from build123d import *

# Parameters (mm, degrees)
SKETCH_1_W          = 40
SKETCH_1_H          = 20
EXTRUDE_1_DEPTH     = 149.5
SKETCH_2_W          = 38
SKETCH_2_H          = 18
CUT_EXTRUDE_1_DEPTH = 2999
SKETCH_4_R          = 2.05
CUT_EXTRUDE_2_DEPTH = 2999
SKETCH_5_R          = 2.025
CUT_EXTRUDE_3_DEPTH = 2999
CUT_EXTRUDE_START   = -21
SKETCH_6_R          = 1.525
CUT_EXTRUDE_4_DEPTH = 22
CUT_EXTRUDE_START_2 = -41
SKETCH_8_R          = 1.525
CUT_EXTRUDE_5_DEPTH = 42


with BuildPart() as part:
    # 草图1 → 凸台-拉伸1 (new body, symmetric)
    with BuildSketch(Plane(origin=(0, 0, 0), x_dir=(0, 0, -1), z_dir=(1, 0, 0))):
        Rectangle(SKETCH_1_W, SKETCH_1_H)
    extrude(amount=EXTRUDE_1_DEPTH, both=True)

    # 草图2 → 切除-拉伸1 (cut)
    with BuildSketch(Plane.ZY.offset(149.5)):
        Rectangle(SKETCH_2_W, SKETCH_2_H)
    extrude(amount=-CUT_EXTRUDE_1_DEPTH, mode=Mode.SUBTRACT)

    # 草图4 → 切除-拉伸2 (cut)
    with BuildSketch(Plane(origin=(0, 10, 0), x_dir=(1, 0, 0), z_dir=(0, 1, 0))):
        with Locations((-47.5, 12.5)):
            Circle(SKETCH_4_R)
        with Locations((-47.5, -12.5)):
            Circle(SKETCH_4_R)
        with Locations((47.5, 12.5)):
            Circle(SKETCH_4_R)
        with Locations((47.5, -12.5)):
            Circle(SKETCH_4_R)
    extrude(amount=-CUT_EXTRUDE_2_DEPTH, mode=Mode.SUBTRACT)

    # 草图5 → 切除-拉伸3 (cut)
    with BuildSketch(Plane.XZ.offset(10)):
        with Locations((-125.5, 14)):
            Circle(SKETCH_5_R)
        with Locations((-125.5, -14)):
            Circle(SKETCH_5_R)
        with Locations((-143.5, -14)):
            Circle(SKETCH_5_R)
        with Locations((-143.5, 14)):
            Circle(SKETCH_5_R)
    cut_extrude_3 = extrude(amount=-CUT_EXTRUDE_3_DEPTH, mode=Mode.SUBTRACT)

    # 镜向1: 切除-拉伸3 across plane
    add(cut_extrude_3.mirror(Plane(origin=(0, 0, 0), x_dir=(0, 0, 1), z_dir=(1, 0, 0))), mode=Mode.SUBTRACT)

    # 草图6 → 切除-拉伸4 (cut)
    with BuildSketch(Plane(origin=(0, 10, 0), x_dir=(1, 0, 0), z_dir=(0, 1, 0)).offset(CUT_EXTRUDE_START)):
        with Locations((-97.25, 16)):
            Circle(SKETCH_6_R)
        with Locations((-97.25, -16)):
            Circle(SKETCH_6_R)
        with Locations((-77.25, -16)):
            Circle(SKETCH_6_R)
        with Locations((-77.25, 16)):
            Circle(SKETCH_6_R)
    cut_extrude_4 = extrude(amount=CUT_EXTRUDE_4_DEPTH, mode=Mode.SUBTRACT)

    # 草图8 → 切除-拉伸5 (cut)
    with BuildSketch(Plane.XY.offset(20).offset(CUT_EXTRUDE_START_2)):
        with Locations((-107.25, 6)):
            Circle(SKETCH_8_R)
        with Locations((-87.25, 6)):
            Circle(SKETCH_8_R)
    cut_extrude_5 = extrude(amount=CUT_EXTRUDE_5_DEPTH, mode=Mode.SUBTRACT)

    # 镜向2: 切除-拉伸4, 切除-拉伸5 across plane
    add(cut_extrude_4.mirror(Plane(origin=(0, 0, 0), x_dir=(0, 0, 1), z_dir=(1, 0, 0))), mode=Mode.SUBTRACT)
    add(cut_extrude_5.mirror(Plane(origin=(0, 0, 0), x_dir=(0, 0, 1), z_dir=(1, 0, 0))), mode=Mode.SUBTRACT)


solid = part.part
Could you check a few things on this model? Use its own coordinates, in mm. A direction names the side the tool comes from. Give positions to 0.01 mm unless a question says otherwise; leave off trailing zeros. Loops run counter-clockwise (first coordinate to the right, second up) from the corner with the lowest first, then second, coordinate; pieces in that order, holes last. Notation, with made-up numbers: (9.5, 33) -> (53.5, 33) arc R17 ccw to (53.5, 48) -> close; hole circle Ø4 at (-33.5, 24.25). An arc over 180 degrees is marked (long way). Return JSON: item names as keys, results as strings.
Item 1: If we section it at C-C on x = 31: List the corners of the cut face in (y, z) for me.
Geometry results:
{"outline": "(-10, -20) -> (10, -20) -> (10, 20) -> (-10, 20) -> close; hole (-9, -19) -> (9, -19) -> (9, 19) -> (-9, 19) -> close"}
Item 2: If we section it at B-B on z = -7: List the corners of the cut face in (x, y) for me.
Geometry results:
{"outline": "(-149.5, -10) -> (149.5, -10) -> (149.5, -9) -> (-149.5, -9) -> close; (-149.5, 9) -> (149.5, 9) -> (149.5, 10) -> (-149.5, 10) -> close"}
Item 3: I need wall thicknesses on L1, parallel to Z at x = -47.5, y = -9.25; L2, parallel to Z at x = -125.5, y = -9.45 (3 decimals); L3, parallel to Y at x = -83.5, z = -10.5. Which ranges of each line are inside material? Lowest first, please. Write a range as from..to.
Geometry results:
{"L1": "z = -20..-14.55, -10.45..10.45, 14.55..20", "L2": "z = -20..-16.025, -11.975..11.975, 16.025..20", "L3": "y = -10..-9, 9..10"}
Item 4: If we section it at A-A on y = -6: List the corners of the cut face in (x, z) for me.
Geometry results:
{"outline": "(-149.5, -20) -> (149.5, -20) -> (149.5, -19) -> (-149.5, -19) -> close; (-149.5, 19) -> (149.5, 19) -> (149.5, 20) -> (-149.5, 20) -> close"}
Item 5: We'd pull the mould along Y, two halves only. Please class faces 3 (the flat face through (-2, -9, 0)), 4 (the flat face through (2, 0, -20)), 5 (the flat face through (2, 10, 0)), 6 (the flat face through (2, -10, 0)): +Y half, -Y half, draft (parallel to the pull), parting line (faces both ways), or undercut.
Geometry results:
{"face 3": "undercut", "face 4": "draft", "face 5": "+Y half", "face 6": "-Y half"}
Item 6: Which directions (+Z, -Z, +X, -X, +Y, -Y) give clear straight access to the entire face, cutting with the end or side of a thin tool? Please do faces 1 (the flat face through (-2, 9, 0)), 2 (the flat face through (149.5, -9.6, 1.6)).
Geometry results:
{"face 1": "+X, -X", "face 2": "+Z, -Z, +X, +Y, -Y"}
